Check sheet for the modelled part. Datum: model origin and axes. Units: mm. Coordinates: 2 decimals unless noted, no trailing zeros. Loops run counter-clockwise (first coordinate to the right, second up) from the corner with the lowest first, then second, coordinate; pieces in that order, holes last. Notation, with made-up numbers: M -24.5,66.25 L -19.5,66.25 A29 ccw -19.5,86.25 Z; hole C 45,9.5 d7. An arc over 180 degrees is marked long. Return JSON: item names as keys, results as strings.
from build123d import *

# Parameters (mm, degrees)
F0_R     = 12
F0_R_2   = 7.5
F1_DEPTH = 73
F2_SIZE  = 0.25
F3_SIZE  = 0.75


with BuildPart() as f1:
    # F0 (on Front) → F1 (new body)
    with BuildSketch(Plane.XZ):
        Circle(F0_R)
        Circle(F0_R_2, mode=Mode.SUBTRACT)
    extrude(amount=F1_DEPTH)

    # F2
    f2_edges = [f1.edges().sort_by_distance(p)[0] for p in [
        (-12, -73, 0),
        (-12, 0, 0),
    ]]
    chamfer(f2_edges, length=F2_SIZE)

    # F3
    f3_edges = [f1.edges().sort_by_distance(p)[0] for p in [
        (-7.5, -73, 0),
        (-7.5, 0, 0),
    ]]
    chamfer(f3_edges, length=F3_SIZE)


solid = f1.part
1) Section check C-C on y = -66. Record the cut outline in (x, z), then the cut area to 3 significant figures.
Answers:
{"outline": "C 0,0 d24; hole C 0,0 d15", "area": "276 mm²"}
2) Section check B-B on x = 0. Record the cut outline in (y, z), then the cut area to 3 significant figures.
Answers:
{"outline": "M -73,-11.75 L -72.75,-12 L -0.25,-12 L 0,-11.75 L 0,-8.25 L -0.75,-7.5 L -72.25,-7.5 L -73,-8.25 Z; M -73,8.25 L -72.25,7.5 L -0.75,7.5 L 0,8.25 L 0,11.75 L -0.25,12 L -72.75,12 L -73,11.75 Z", "area": "656 mm²"}
3) Go/stop test with flat-tipped pins: pin 1 Ø1.5 at (x, y) = (5, -42.5) entering from +Z; pin 2 Ø2 at (y, z) = (-52, -6) entering from +X; pin 3 Ø5 at (y, z) = (-55, 7) entering from +X; pin 4 Ø12 at (x, z) = (0, 0) entering from +Y. Record where each tip stops, or that it passes through.
Answers:
{"pin 1": "z = 11.22", "pin 2": "x = 10.91", "pin 3": "x = 11.12", "pin 4": "through"}
4) Scan lines: line 1 along Z through (x, y) = (0, -17); line 2 along X through (y, z) = (-55, 5.5); line 3 along Z through (x, y) = (-2.25, -57). Record each from-to range of solid material in increasing order. Write a range as [from, to].
Answers:
{"line 1": "[-12, -7.5], [7.5, 12]", "line 2": "[-10.67, -5.1], [5.1, 10.67]", "line 3": "[-11.79, -7.15], [7.15, 11.79]"}
5) Section check A-A on z = 0. Record the cut outline in (x, y), then the cut area to 3 significant figures.
Answers:
{"outline": "M -12,-72.75 L -11.75,-73 L -8.25,-73 L -7.5,-72.25 L -7.5,-0.75 L -8.25,0 L -11.75,0 L -12,-0.25 Z; M 7.5,-72.25 L 8.25,-73 L 11.75,-73 L 12,-72.75 L 12,-0.25 L 11.75,0 L 8.25,0 L 7.5,-0.75 Z", "area": "656 mm²"}
6) Draft check along Z on faces 1 (the face through (-8, -73, 3)), 2 (the face through (-11.99, -35.99, 0.53)), 3 (the face through (-7.493, -36, 0.33)). Enter one of: +Z half, -Z half, draft (parallel to the pull), parting line (faces both ways), or undercut.
Answers:
{"face 1": "draft", "face 2": "parting line", "face 3": "undercut"}
